The listing builds one solid part. Answer for the finished solid, in the listing's coordinates (mm). Face numbers are marked on the shaded views. A direction names the side the tool comes from. Give positions to 0.01 mm unless a question says otherwise; leave off trailing zeros. Loops run counter-clockwise (first coordinate to the right, second up) from the corner with the lowest first, then second, coordinate; pieces in that order, holes last. Notation, with made-up numbers: M 42.25,48.5 L 70.25,48.5 A20 cw 70.25,72.5 Z; hole C -30.75,69.25 d2. An arc over 180 degrees is marked long. Return JSON: item names as keys, results as strings.
from build123d import *

# Parameters (mm, degrees)
F0_R     = 2.5
F1_DEPTH = 2


# Not quite as in the source:
# - a feature names something its author has since deleted; it is built from what else it names


with BuildPart() as f1:
    # F0 (on Front) → F1 (new body, symmetric)
    with BuildSketch(Plane.XZ):
        with BuildLine():
            Line((4.5, 4.5), (0, 4.5))
            ThreePointArc((0, 4.5), (-4.5, 0), (0, -4.5))
            Line((0, -4.5), (4.5, -4.5))
            Line((4.5, -4.5), (4.5, 0))
            Line((4.5, 0), (4.5, 4.5))
        make_face()
        Circle(F0_R, mode=Mode.SUBTRACT)
    extrude(amount=F1_DEPTH, both=True)

    # F0 (on Front) → F2 (revolve)
    with BuildSketch(Plane.XZ):
        Polygon((4.5, 8), (4.5, 4.5), (4.5, 0), (57.5, 0), (57.5, 5.5), (49.5, 6.5), (14.5, 6.5), (14.5, 9), (11, 9), (11, 8), align=None)
    revolve(axis=Axis((31, 0, 0), (1, 0, 0)))


solid = f1.part
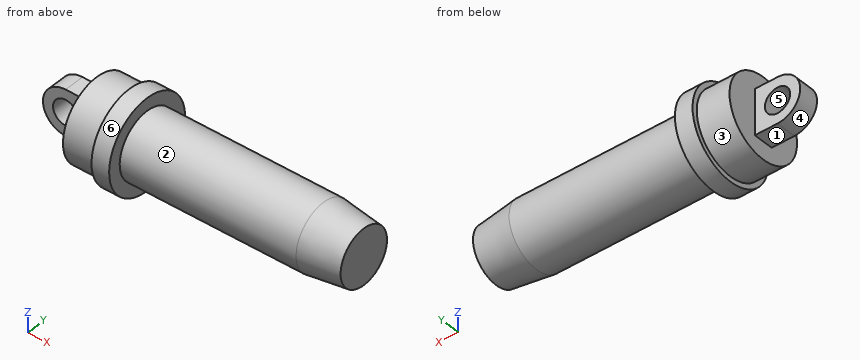
(1) The part is cut by section C-C (x = 12.5). Determine the outline of the cut face in (y, z), and give its area (3 significant figures).
Values follow:
{"outline": "C 0,0 d18", "area": "254 mm²"}
(2) Straight lines are drawn through the part: line 1 along X through (y, z) = (7, -4.5); line 2 along X through (y, z) = (0.5, -2.25); line 3 along X through (y, z) = (-3.25, -4). For each, find the intervals that lie inside material, in ascending order.
Values follow:
{"line 1": "11 to 14.5", "line 2": "-3.9 to -1.09, 1.09 to 57.5", "line 3": "4.5 to 57.5"}
(3) Determine the mould class of the marked faces 4, 5 and 6 for opening direction X: released by +X, released by -X, zero draft, split by the parting line, or undercut.
Values follow:
{"face 4": "released by -X", "face 5": "undercut", "face 6": "zero draft"}
(4) The part is cut by section D-D (x = 47.5). Determine the outline of the cut face in (y, z).
Values follow:
{"outline": "C 0,0 d13"}
(5) Given pin 1 (3 mm diameter, centred on y = 1, z = 4, fed in from -X); pin 2 (6 mm diameter, centred on x = 9.5, z = -6.5, fed in from -Y); pin 3 (4 mm diameter, centred on x = 49, z = -6.5, fed in from -Y), each flat-ended and moving along its own axis, determine where each tip first touches the part or whether it passes through.
Values follow:
{"pin 1": "x = -3.74", "pin 2": "y = -8.11", "pin 3": "y = -4.69"}
(6) A tool of negligible diameter and unlimited length cuts with its end or side. For the marked faces 1, 2 and 3, from which of +Z, -Z, +X, -X, +Y, -Y can it reach the whole face along a straight path? Write none if from no direction.
Values follow:
{"face 1": "-Z, -X, +Y, -Y", "face 2": "+X", "face 3": "-X"}
(7) The part is cut by section B-B (y = 0). Determine the outline of the cut face in (x, z).
Values follow:
{"outline": "M 0,-4.5 L 4.5,-4.5 L 4.5,-8 L 11,-8 L 11,-9 L 14.5,-9 L 14.5,-6.5 L 49.5,-6.5 L 57.5,-5.5 L 57.5,5.5 L 49.5,6.5 L 14.5,6.5 L 14.5,9 L 11,9 L 11,8 L 4.5,8 L 4.5,4.5 L 0,4.5 A4.5 ccw Z; hole C 0,0 d5"}
(8) The part is cut by section A-A (z = 0). Determine the outline of the cut face in (x, y).
Values follow:
{"outline": "M -4.5,-2 L -2.5,-2 L -2.5,2 L -4.5,2 Z; M 2.5,-2 L 4.5,-2 L 4.5,-8 L 11,-8 L 11,-9 L 14.5,-9 L 14.5,-6.5 L 49.5,-6.5 L 57.5,-5.5 L 57.5,5.5 L 49.5,6.5 L 14.5,6.5 L 14.5,9 L 11,9 L 11,8 L 4.5,8 L 4.5,2 L 2.5,2 Z"}
